from build123d import *

# Parameters (mm, degrees)
F0_W     = 66.776178
F0_H     = 12.991002
F1_DEPTH = 10.922
F2_W     = 18.454506
F2_H     = 7.770319
F3_DEPTH = 10.414
F4_R     = 4.070445
F5_DEPTH = 37.846
F6_W     = 16.026282
F6_H     = 4.97786
F7_DEPTH = 10.414


with BuildPart() as f1:
    # F0 (on Front) → F1 (new body)
    with BuildSketch(Plane.XZ):
        with Locations((2.792459, 6.495501)):
            Rectangle(F0_W, F0_H)
        Polygon((-15.054992, 30.231398), (-30.59563, 12.991002), (36.180548, 12.991002), (18.940151, 30.231398), align=None)
    extrude(amount=-F1_DEPTH)

    # F2 (on Front) → F3 (join)
    with BuildSketch(Plane.XZ):
        with Locations((1.214112, 26.103414)):
            Rectangle(F2_W, F2_H)
    extrude(amount=F3_DEPTH)

    # F4 (on Top) → F5 (cut)
    with BuildSketch(Plane.XY):
        with Locations((1.699758, -4.97786)):
            Circle(F4_R)
    extrude(amount=F5_DEPTH, mode=Mode.SUBTRACT)

    # F6 (on Front) → F7 (join)
    with BuildSketch(Plane.XZ):
        with Locations((1.214112, 2.48893)):
            Rectangle(F6_W, F6_H)
        Polygon((-3.399515, 9.105843), (-6.799029, 4.97786), (9.227253, 4.97786), (5.827739, 9.105843), align=None)
    extrude(amount=F7_DEPTH)


solid = f1.part
Work out the finished part from the listing and answer in its coordinate system (mm). A direction names the side the tool comes from. Round coordinates to 2 decimals unless told otherwise and drop trailing zeros. Write each loop counter-clockwise with the first axis right and the second up, starting at its lowest first coordinate (ties: lowest second). Pieces come first, ordered by that corner, then holes.
1) The mould has two halves that part along Z. Classify faces 5 (the flat face through (2, 5, 30.231)), 6 (the flat face through (-5.075, -5.134, 7.071)), 7 (the flat face through (2, 10.922, 15)): pulls with the +Z half, pulls with the -Z half, needs draft (parallel to the pull), parting line crosses it, or undercut.
2) A tool of negligible diameter and unlimited length cuts with its end or side. For faces 1 (the flat face through (-3, -5, 29.989)), 2 (the cylindrical face through (1.17, -0.942, 26.049)), 3 (the flat face through (-8.013, -5, 26)), 4 (the flat face through (7.551, -5.134, 7.013)), from which of +Z, -Z, +X, -X, +Y, -Y can it reach the whole face along a straight path? Write none if from no direction.
3) A cutting plane is placed at A-A (y = -7). Give the vertices of the cut face in (x, z), plus the area to 3 significant figures.
4) A cutting plane is placed at B-B (x = 2.5). Give the vertices of the cut face in (y, z), plus the area to 3 significant figures.
5) Given pin 1 Ø1.5 at (y, z) = (-4, 2.5) entering from +X; pin 2 Ø8.5 at (y, z) = (-7.5, 28) entering from -X; pin 3 Ø3 at (y, z) = (-7, 19.5) entering from -X; pin 4 Ø5 at (x, z) = (25.5, 23) entering from -Y, each flat-ended and moving along its own axis, determine where each tip first touches the part or whether it passes through.
6) A cutting plane is placed at D-D (z = 10.5). Give the vertices of the cut face in (x, y).
7) Straight lines are drawn through the part: line 1 (Y direction, x = -24.5, z = 2); line 2 (X direction, y = -9.5, z = 23); line 3 (Y direction, x = 3.5, z = 29). For each, find the intervals that lie inside material, in ascending order.
8) A cutting plane is placed at C-C (y = 7.75). Give the vertices of the cut face in (x, z) (3 decimals).
Completed:
1. face 5: pulls with the +Z half
1. face 6: undercut
1. face 7: needs draft
2. face 1: +Z, +X, -X, -Y
2. face 2: +Z
2. face 3: +Z, -Z, -X, -Y
2. face 4: +X, -Y
3. outline: (-8.01, 22.22) - (-1.83, 22.22) - (-1.83, 29.99) - (-8.01, 29.99) - close; (-6.8, 0) - (9.23, 0) - (9.23, 4.98) - (5.83, 9.11) - (-3.4, 9.11) - (-6.8, 4.98) - close; (5.23, 22.22) - (10.44, 22.22) - (10.44, 29.99) - (5.23, 29.99) - close
3. area: 220 mm2
4. outline: (-10.41, 0) - (10.92, 0) - (10.92, 30.23) - (0, 30.23) - (0, 29.99) - (-0.99, 29.99) - (-0.99, 22.22) - (0, 22.22) - (0, 9.11) - (-10.41, 9.11) - close; (-10.41, 22.22) - (-8.97, 22.22) - (-8.97, 29.99) - (-10.41, 29.99) - close
4. area: 444 mm2
5. pin 1: stops at x = 9.23
5. pin 2: stops at x = -8.01
5. pin 3: passes through
5. pin 4: stops at y = 0
6. outline: (-30.6, 0) - (36.18, 0) - (36.18, 10.92) - (-30.6, 10.92) - close
7. line 1: y = 0 to 10.92
7. line 2: x = -8.01 to 10.44
7. line 3: y = -10.41 to -8.63, -1.33 to 10.92
8. outline: (-30.596, 0) - (36.181, 0) - (36.181, 12.991) - (18.94, 30.231) - (-15.055, 30.231) - (-30.596, 12.991) - close
